from build123d import *

# Parameters (mm, degrees)
CUT_EXTRUDE1_REACH = 53.886
CIRPATTERN1_COUNT  = 8


with BuildPart() as part:
    # Sketch1 → Revolve1 (revolve)
    with BuildSketch(Plane(origin=(0, 0, 0), x_dir=(0, 0, -1), z_dir=(1, 0, 0)), mode=Mode.PRIVATE) as revolve1_sk:
        Polygon((-8.89, 1.27), (3.81, 1.27), (3.81, 6.35), (13.97, 25.4), (13.97, 31.75), (11.43, 31.75), (11.43, 29.21), (-9.49, 29.21), (-9.49, 31.75), (-12.03, 31.75), (-12.03, 25.4), (-3.81, 6.35), (-8.89, 4.445), align=None)
    revolve(revolve1_sk.sketch.rotate(Axis((0, 0, 0), (0, 0, -1)), 90), axis=Axis((0, 0, 0), (0, 0, -1)))

    # Cut-Extrude1: up to this cone (the profile starts outside it)
    cut_extrude1_end = Plane(origin=(0, 0, 12.03), z_dir=(0, 0, -1)).offset(12.453334333) * Cone(1.875e-06, 78.62375, 41.932665667, align=(Align.CENTER, Align.CENTER, Align.MIN), mode=Mode.PRIVATE)
    # Sketch2 → Cut-Extrude1 (cut, up to the surface)
    with BuildSketch(Plane.XY.offset(12.03), mode=Mode.PRIVATE) as cut_extrude1_sk1:
        with BuildLine():
            Line((-5.259202996, 19.62761279), (-1.643500936, 6.133628997))
            ThreePointArc((-1.643500936, 6.133628997), (0, 6.35), (1.643500936, 6.133628997))
            Line((1.643500936, 6.133628997), (5.259202996, 19.62761279))
            ThreePointArc((5.259202996, 19.62761279), (0, 20.32), (-5.259202996, 19.62761279))
        make_face()
    cut_extrude1_tool1 = extrude(cut_extrude1_sk1.sketch, amount=-CUT_EXTRUDE1_REACH, mode=Mode.PRIVATE) - cut_extrude1_end
    cut_extrude1 = cut_extrude1_tool1.solids().sort_by_distance((0, 14.388913, 12.03))[0]
    add(cut_extrude1, mode=Mode.SUBTRACT)

    # CirPattern1: Cut-Extrude1 ×8 about axis
    cirpattern1_axis = Axis((0, 0, 0), (0, 0, 1))
    for i in range(1, CIRPATTERN1_COUNT):
        add(cut_extrude1.rotate(cirpattern1_axis, i * 360 / CIRPATTERN1_COUNT), mode=Mode.SUBTRACT)


solid = part.part
Build history of the part. All positions in model axes, mm. A direction names the side the tool comes from. Coordinates: 2 decimals unless noted, no trailing zeros. One line per question, with ' | ' between items. Start each with the question number.
Q1. Probe L1, parallel to Y at x = 0, z = 0.25; L2, parallel to Z at x = -15, y = 26; L3, parallel to X at y = 1, z = 5.25. List the from-to ranges inside material, lowest first. Write a range as from..to.
Q2. Two-plate mould, pull along Z, no slides. Class faces 4 (the face through (-26, 14, 9.49)), 5 (the face through (14, 26, -11.43)), 6 (the face through (-4.47, -4.51, 0.05)), 7 (the face through (6.72, 2.79, 4.21)): +Z half, -Z half, draft (parallel to the pull), parting line (faces both ways), or undercut.
Q3. 3-axis set-ups, long thin cutter, end or side, ignore diameter. For faces 1 (the face through (4.53, -1.43, 8.08)), 2 (the face through (4.51, -4.47, 0.05)), 3 (the face through (1.5, -0.1, -3.81)): which of +Z, -Z, +X, -X, +Y, -Y reach the whole face in a straight line?
Q4. Flat gauge pins, fed straight in: pin 1 Ø1 at (x, z) = (5.5, -6.5) entering from -Y; pin 2 Ø5 at (y, z) = (20, 2) entering from +X; pin 3 Ø2 at (x, y) = (0, 0) entering from +Z; pin 4 Ø12 at (x, y) = (-1, 9.5) entering from -Z. Where does each tip first touch, or does it go through?
Q5. Saw through at A-A (x = 0). Count the separate pieces of the cut face and the enclosed holes in it, then the cut area to 3 significant figures.
Check values:
1) L1: y = -29.21..-20.32, -6.35..-1.27, 1.27..6.35, 20.32..29.21 | L2: z = -13.97..-11.43, 9.49..12.03 | L3: x = -29.19..-20.3, -5.72..-0.78, 0.78..5.72, 20.3..29.19
2) face 4: undercut | face 5: undercut | face 6: draft | face 7: +Z half
3) face 1: +Z | face 2: +Z, -Z | face 3: -Z
4) pin 1: stops at y = -28.78 | pin 2: stops at x = 23.39 | pin 3: passes through | pin 4: stops at z = -8.55
5) separate pieces: 4 | enclosed holes: 0 | area: 583 mm2
